Part model, mm, in its own coordinate system. A direction names the side the tool comes from. Round coordinates to 2 decimals unless told otherwise and drop trailing zeros. Write each loop counter-clockwise with the first axis right and the second up, starting at its lowest first coordinate (ties: lowest second). Pieces come first, ordered by that corner, then holes.
from build123d import *

# Parameters (mm, degrees)
F1_DEPTH = 254
F2_R     = 6.35
F3_DEPTH = 39.0204481418
F4_W     = 76.2
F4_H     = 22.7825300816
F5_DEPTH = 101.6
F9_R     = 19.05
F10_SIZE = 5.08


with BuildPart() as f1:
    # F0 (on Front) → F1 (new body)
    with BuildSketch(Plane.XZ):
        Polygon((-19.1467776895, 28.3457897604), (16.7935416102, -16.5796130896), (19.7885707021, 25.7786232978), align=None)
    extrude(amount=F1_DEPTH)

    # F2 (on face) → F3 (cut, through all)
    with BuildSketch(Plane(origin=(17.876465035, 0, -1.263993438), x_dir=(0, 1, 0), z_dir=(0.9975095855, 0, -0.0705310344))):
        with Locations((-127, 10.0461428802)):
            Circle(F2_R)
    extrude(amount=-F3_DEPTH, mode=Mode.SUBTRACT)

    # F4 (on face) → F5 (join)
    with BuildSketch(Plane(origin=(17.876465035, 0, -1.263993438), x_dir=(0, 1, 0), z_dir=(0.9975095855, 0, -0.0705310344))):
        with Locations((-173.4407693148, 0.2275721636)):
            Rectangle(F4_W, F4_H)
    extrude(amount=F5_DEPTH)

    # F7 (on offset) → F8 (revolve, cut)
    with BuildSketch(Plane(origin=(0, -186.1407693148, 0), x_dir=(-1, 0, 0), z_dir=(0, 1, 0))):
        Polygon((-91.9674258711, 0), (-91.5099222483, -6.4704034611), (-39.0226445365, -2.7591789837), (-41.141692549, 6.2215458602), (-67.5091892481, 0), align=None)
    revolve(axis=Axis((56.3993897732, -186.1407693148, -3.9878386717), (0.9975095855, 0, -0.0705310344)), mode=Mode.SUBTRACT)

    # F9
    f9_edges = [f1.edges().sort_by_distance(p)[0] for p in [
        (69.369441, -135.340769, 6.742931),
        (69.369441, -211.540769, 6.742931),
        (0.320897, -254, 27.062207),
    ]]
    fillet(f9_edges, radius=F9_R)

    # F10
    f10_edges = [f1.edges().sort_by_distance(p)[0] for p in [
        (0.320897, 0, 27.062207),
    ]]
    chamfer(f10_edges, length=F10_SIZE)


solid = f1.part
Q1. Tool access for faces 4 (the conical face through (39.134, -185.635, -2.503)), 5 (the flat face through (0.593, -118.406, 27.044)), 6 (the flat face through (67.053, -173.974, -15.933)): list every direction of +Z, -Z, +X, -X, +Y, -Y with a clear straight run to the whole face (end or side of a thin tool).
Q2. Saw through at B-B, the plane y = -114.5. Write the cut outline in (x, z), and give its area (3 significant figures).
Q3. Drop flat-ended pins along their axis: P1, Ø5.5, axis at x = 65.5, z = -12.5, coming from the +Y side; P2, Ø2, axis at x = 15, z = 17, coming from the -Y side; P3, Ø8.5, axis at x = 93, z = -14, coming from the -Y side. Give the stop position or say it passes through.
Q4. Saw through at A-A, the plane y = -164.5. Write the cut outline in (x, z).
Q5. Wall check: line 1 (Y direction, x = 86, z = -14.5); line 2 (Y direction, x = 18.5, z = 11.5); line 3 (Y direction, x = 95, z = -3). Give the ranges that are in metal, low to high.
Q6. Two-plate mould, pull along Y, no slides. Class faces 1 (the flat face through (10, -254, 1)), 2 (the cylindrical face through (7.8, -123.59, 14.89)), 3 (the flat face through (0.42, -2.5, 24.47)): released by +Y, released by -Y, zero draft, split by the parting line, or undercut.
Computed:
1. face 4: none
1. face 5: +Z, +X, +Y, -Y
1. face 6: -Z, +Y, -Y
2. outline: (-19.15, 28.35) - (16.79, -16.58) - (19.79, 25.78) - close
2. area: 828 mm2
3. P1: stops at y = -135.34
3. P2: stops at y = -251.75
3. P3: stops at y = -211.54
4. outline: (-19.15, 28.35) - (16.79, -16.58) - (17.09, -12.4) - (118.44, -19.57) - (120.04, 3.16) - (18.7, 10.33) - (19.79, 25.78) - close
5. line 1: y = -211.54 to -135.34
5. line 2: y = -253.41 to -132.73, -121.27 to 0
5. line 3: y = -207.94 to -138.94
6. face 1: released by -Y
6. face 2: undercut
6. face 3: released by +Y
